```python
from build123d import *

# Parameters (mm, degrees)
SKETCH1_W           = 76.2
SKETCH1_H           = 38.1
BOSS_EXTRUDE1_DEPTH = 2.54
SKETCH2_W           = 15.24
SKETCH2_H           = 7.747
SKETCH2_W_2         = 30.48
SKETCH2_W_3         = 38.1
BOSS_EXTRUDE2_DEPTH = 6.35
SKETCH3_W           = 8.89
SKETCH3_H           = 21.59
CUT_EXTRUDE1_DEPTH  = 6.08
SKETCH4_W           = 12.7
SKETCH4_H           = 6.35
CUT_EXTRUDE2_DEPTH  = 7.747
SKETCH5_R           = 3.175
CUT_EXTRUDE3_DEPTH  = 12.43


with BuildPart() as part:
    # Sketch1 → Boss-Extrude1 (new body, symmetric)
    with BuildSketch(Plane(origin=(0, 0, 0), x_dir=(1, 0, 0), z_dir=(0, 1, 0))):
        Rectangle(SKETCH1_W, SKETCH1_H)
    extrude(amount=BOSS_EXTRUDE1_DEPTH, both=True)

    # Sketch2 → Boss-Extrude2 (add)
    with BuildSketch(Plane(origin=(0, 2.54, 0), x_dir=(1, 0, 0), z_dir=(0, 1, 0))):
        with Locations((-30.48, 15.1765)):
            Rectangle(SKETCH2_W, SKETCH2_H)
        with Locations((22.86, 15.1765)):
            Rectangle(SKETCH2_W_2, SKETCH2_H)
        with Locations((19.05, -15.1765)):
            Rectangle(SKETCH2_W_3, SKETCH2_H)
        with Locations((-30.48, -15.1765)):
            Rectangle(SKETCH2_W, SKETCH2_H)
    extrude(amount=BOSS_EXTRUDE2_DEPTH)

    # Sketch3 → Cut-Extrude1 (cut, through all)
    with BuildSketch(Plane(origin=(0, 2.54, 0), x_dir=(1, 0, 0), z_dir=(0, 1, 0))):
        with Locations((-17.145, 8.255)):
            Rectangle(SKETCH3_W, SKETCH3_H)
    extrude(amount=-CUT_EXTRUDE1_DEPTH, mode=Mode.SUBTRACT)

    # Sketch4 → Cut-Extrude2 (cut)
    with BuildSketch(Plane.XY.offset(19.05)):
        with Locations((31.75, 5.715)):
            Rectangle(SKETCH4_W, SKETCH4_H)
    extrude(amount=-CUT_EXTRUDE2_DEPTH, mode=Mode.SUBTRACT)

    # Sketch5 → Cut-Extrude3 (cut, through all)
    with BuildSketch(Plane.XZ.offset(2.54)):
        with Locations((25.4, 6.35)):
            Circle(SKETCH5_R)
        with Locations((-31.75, 0)):
            Circle(SKETCH5_R)
    extrude(amount=-CUT_EXTRUDE3_DEPTH, mode=Mode.SUBTRACT)


solid = part.part
```
Build history of the part. All positions in model axes, mm. A direction names the side the tool comes from. Give positions to 0.01 mm unless a question says otherwise; leave off trailing zeros. Order: outer loops, then holes, each group sorted by start corner. A loop starts at its lowest first (then second) coordinate and runs counter-clockwise, first axis right, second up. Notation, with made-up numbers: M 14,55.5 L 53,55.5 A24 ccw 53,83.5 Z; hole C -25.75,26.5 d7. An arc over 180 degrees is marked long. Write item = value, one per line. Start each with the question number.
(1) Slice it at A-A on z = 6.35. Write the cut outline in (x, y) (3 decimals).
(2) Probe L1, parallel to X at y = -0.5, z = -5.5; L2, parallel to X at y = 4, z = -13; L3, parallel to Z at x = -29.5, y = 8.25. List the from-to ranges inside material, lowest first. Write a range as [from, to].
(3) Slice it at D-D on z = 16.5. Write the cut outline in (x, y).
(4) Slice it at C-C on y = 1. Write the cut outline in (x, z) (3 decimals), plus the area to 3 significant figures.
(5) Pin check, flat tips, straight feed: pin 1 Ø5 at (x, y) = (-7.5, 7.5) entering from -Z; pin 2 Ø2.5 at (x, y) = (-15.5, 0.5) entering from -Z; pin 3 Ø11.5 at (x, z) = (11.5, -1) entering from +Y; pin 4 Ø1.5 at (y, z) = (5, 11.5) entering from +X. Stop position of each tip, or through.
(6) Two-plate mould, pull along X, no slides. Class faces 1 (the flat face through (-22.86, 6, -15)), 2 (the flat face through (13, 6, 11.303)), 3 (the flat face through (-38.1, 2, 0)), 4 (the flat face through (-22.86, 6, 15)): released by +X, released by -X, zero draft, split by the parting line, or undercut.
(7) Slice it at B-B on x = -31.75. Write the cut outline in (y, z) (3 decimals).
(8) Which spindle directions (+Z, -Z, +X, -X, +Y, -Y) get a long thin tool onto all of the face, cutting with end or side? Do faces 5 (the flat face through (-21.59, 0, -8)), 6 (the flat face through (7.62, 6, -15)), 7 (the flat face through (-31, 6, 11.303)), 8 (the flat face through (25.4, 6, 15)). Say none if no direction does.
Responses:
q1.outline = M -38.1,-2.54 L 22.225,-2.54 L 22.225,2.54 L -38.1,2.54 Z; M 28.575,-2.54 L 38.1,-2.54 L 38.1,2.54 L 28.575,2.54 Z
q2.L1 = [-38.1, -21.59], [-12.7, 38.1]
q2.L2 = [-38.1, -22.86], [7.62, 38.1]
q2.L3 = [-19.05, -11.3], [11.3, 19.05]
q3.outline = M -38.1,-2.54 L 38.1,-2.54 L 38.1,2.54 L 25.4,2.54 L 25.4,8.89 L 0,8.89 L 0,2.54 L -22.86,2.54 L -22.86,8.89 L -38.1,8.89 Z
q4.outline = M -38.1,-19.05 L -21.59,-19.05 L -21.59,2.54 L -12.7,2.54 L -12.7,-19.05 L 38.1,-19.05 L 38.1,19.05 L -38.1,19.05 Z; hole C -31.75,0 d6.35; hole C 25.4,6.35 d6.35
q4.area = 2,650 mm2
q5.pin_1 = through
q5.pin_2 = 2.54
q5.pin_3 = 2.54
q5.pin_4 = 25.4
q6.face_1 = undercut
q6.face_2 = zero draft
q6.face_3 = released by -X
q6.face_4 = undercut
q7.outline = M -2.54,-19.05 L 8.89,-19.05 L 8.89,-11.303 L 2.54,-11.303 L 2.54,-3.175 L -2.54,-3.175 Z; M -2.54,3.175 L 2.54,3.175 L 2.54,11.303 L 8.89,11.303 L 8.89,19.05 L -2.54,19.05 Z
q8.face_5 = -Z, +Y, -Y
q8.face_6 = -Z, +Y
q8.face_7 = +X, -X, +Y
q8.face_8 = +Z, +X, +Y
